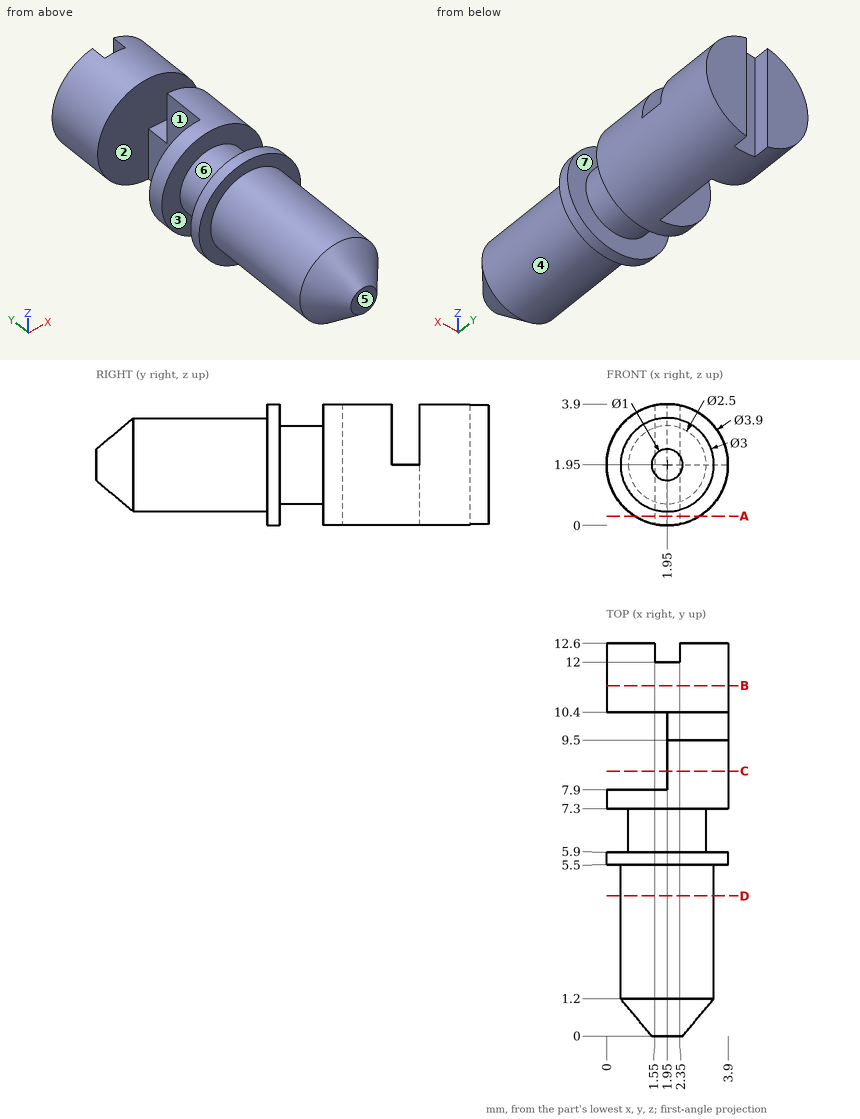
Job drawing, mm, ordinate dimensions from the low corner. One solid piece. A direction names the side the tool comes from. Give positions to 0.01 mm unless a question says otherwise; leave off trailing zeros. Write each loop counter-clockwise with the first axis right and the second up, starting at its lowest first coordinate (ties: lowest second). Pieces come first, ordered by that corner, then holes. Notation, with made-up numbers: M -4,18.25 L 47,18.25 A34 ccw 47,54.25 Z; hole C -14.5,33.5 d10. An arc over 180 degrees is marked long. One line per item, written item: value. Start each with the question number.
Q1. Saw through at D-D, the plane y = 4.5. Write the cut outline in (x, z).
Q2. Probe probe 1 along Y at (x, z) = (1.3, 0.3); probe 2 along Y at (x, z) = (3.5, 2.9); probe 3 along Y at (x, z) = (3.7, 1.55). List the from-to ranges inside material, lowest first. Write a range as [from, to].
Q3. Saw through at A-A, the plane z = 0.3. Write the cut outline in (x, y), plus the area to 3 significant figures.
Q4. Two-plate mould, pull along Y, no slides. Class the marked faces 4, 5, 6 and 7: +Y half, -Y half, draft (parallel to the pull), parting line (faces both ways), or undercut.
Q5. Saw through at C-C, the plane y = 8.5. Write the cut outline in (x, z), plus the area to 3 significant figures.
Q6. Saw through at B-B, the plane y = 11.25. Write the cut outline in (x, z), plus the area to 3 significant figures.
Q7. 3-axis set-ups, long thin cutter, end or side, ignore diameter. For the marked faces 1, 2 and 3: which of +Z, -Z, +X, -X, +Y, -Y reach the whole face in a straight line?
Q8. Drop flat-ended pins along their axis: pin 1 Ø1.2 at (y, z) = (9, 3) entering from -X; pin 2 Ø1.2 at (x, z) = (2, 2) entering from -Y; pin 3 Ø1.5 at (y, z) = (8.5, 3.5) entering from -X. Give the stop position or say it passes through.
Output values:
1. outline: C 1.95,1.95 d3
2. probe 1: y = [5.5, 5.9], [7.3, 7.9], [10.4, 12.6]
2. probe 2: y = [5.5, 5.9], [7.3, 9.5], [10.4, 12.6]
2. probe 3: y = [5.5, 5.9], [7.3, 12.6]
3. outline: M 0.91,5.5 L 2.99,5.5 L 2.99,5.9 L 0.91,5.9 Z; M 0.91,7.3 L 2.99,7.3 L 2.99,12.6 L 2.35,12.6 L 2.35,12 L 1.55,12 L 1.55,12.6 L 0.91,12.6 L 0.91,10.4 L 1.95,10.4 L 1.95,7.9 L 0.91,7.9 Z
3. area: 8.77 mm²
4. face 4: draft
4. face 5: -Y half
4. face 6: undercut
4. face 7: undercut
5. outline: M 1.95,0 A1.95 ccw 1.95,3.9 Z
5. area: 5.97 mm²
6. outline: C 1.95,1.95 d3.9
6. area: 11.9 mm²
7. face 1: +Z, -Z, -X
7. face 2: +Z, -X
7. face 3: none
8. pin 1: stops at x = 1.95
8. pin 2: stops at y = 0
8. pin 3: stops at x = 0.34
